```python
from build123d import *

# Parameters (mm, degrees)
F1_DEPTH = 10
F4_DEPTH = 7.5
F2_R     = 22.5
F5_DEPTH = 10.001
F2_R_2   = 40
F6_DEPTH = 5


with BuildPart() as f1:
    # F0 (on Top) → F1 (new body)
    with BuildSketch(Plane.XY):
        Polygon((43.915, 38.863247), (36.278247, 46.5), (-36.278247, 46.5), (-43.915, 38.863247), (-43.915, -46.5), (43.915, -46.5), align=None)
    extrude(amount=F1_DEPTH)

    # F3 (on face) → F4 (cut)
    with BuildSketch(Plane.XY.offset(10)):
        Polygon((-40, 3.114054), (-40, -46.500151), (-36.5154, -46.500151), (-36.5154, -9.207999), (-34, -9.207999), (-34, 3.114054), align=None)
    extrude(amount=-F4_DEPTH, mode=Mode.SUBTRACT)

    # F2 (on face) → F5 (cut, through all)
    with BuildSketch(Plane.XY.offset(10)):
        with Locations((0, 4)):
            Circle(F2_R)
    extrude(amount=-F5_DEPTH, mode=Mode.SUBTRACT)

    # F2 (on face) → F6 (cut)
    with BuildSketch(Plane.XY.offset(10)):
        with Locations((0, 4)):
            Circle(F2_R_2)
        with BuildLine():
            ThreePointArc((2, 35.686945), (31.75, 4), (2, -27.686945))
            Line((2, -27.686945), (2, -25.15))
            Line((2, -25.15), (-2, -25.15))
            Line((-2, -25.15), (-2, -27.686945))
            ThreePointArc((-2, -27.686945), (-31.75, 4), (-2, 35.686945))
            Line((-2, 35.686945), (-2, 33.15))
            Line((-2, 33.15), (2, 33.15))
            Line((2, 33.15), (2, 35.686945))
        make_face(mode=Mode.SUBTRACT)
    extrude(amount=-F6_DEPTH, mode=Mode.SUBTRACT)


solid = f1.part
```
The model under review builds one solid part; all positions refer to its coordinate system, in mm. A direction names the side the tool comes from. Coordinates: 2 decimals unless noted, no trailing zeros. Write each loop counter-clockwise with the first axis right and the second up, starting at its lowest first coordinate (ties: lowest second). Pieces come first, ordered by that corner, then holes. Notation, with made-up numbers: (12, -27.5) -> (50, -27.5) arc R5 ccw to (50, -19.5) -> close; hole circle Ø1 at (5.25, -8). An arc over 180 degrees is marked (long way). One line per item, written item: value. Start each with the question number.
Q1. Add section D-D, the plane x = -38. Give the boundary of the cut face in (y, z), then the cut area to 3 significant figures.
Q2. Add section A-A, the plane z = 8.75. Give the boundary of the cut face in (x, y) (3 decimals), then the cut area to 3 significant figures.
Q3. The part is to be moulded in two halves that separate along X. For faces 4 (the face through (-43.915, -3, 5)), 5 (the face through (1, 46.5, 5)), 6 (the face through (40.15, 42.63, 4.93)), 7 (the face through (-31.743, 3.33, 7.535)), say which applies: +X half, -X half, draft (parallel to the pull), parting line (faces both ways), or undercut.
Q4. To check wall thickness, follow probe 1 along Y at (x, z) = (0, 8.25); probe 2 along Y at (x, z) = (0, 3.5); probe 3 along X at (y, z) = (-16.5, 9) (3 decimals). State the ranges of each line that lie inside material, in increasing order.
Q5. Add section C-C, the plane y = 2. Give the boundary of the cut face in (x, z) (3 decimals).
Q6. Add section B-B, the plane x = 0. Give the boundary of the cut face in (y, z), then the cut area to 4 significant figures.
Q7. For faces 1 (the face through (-36.515, -28, 6)), 2 (the face through (-2, 34, 8)), 3 (the face through (10.382, -15.961, 5.07)), list the 3-axis set-ups (+Z, -Z, +X, -X, +Y, -Y) from which the entire face can be reached by the end or side of a thin tool; tool diameter is ignored.
Response:
1. outline: (-46.5, 0) -> (44.78, 0) -> (44.78, 10) -> (16.49, 10) -> (16.49, 5) -> (3.11, 5) -> (3.11, 2.5) -> (-46.5, 2.5) -> close
1. area: 474 mm²
2. outline: (-43.915, -46.5) -> (-40, -46.5) -> (-40, 3.114) -> (-39.99, 3.114) arc R40 cw (long way) to (-36.515, -12.329) -> (-36.515, -46.5) -> (43.915, -46.5) -> (43.915, 38.863) -> (36.278, 46.5) -> (-36.278, 46.5) -> (-43.915, 38.863) -> close; (-2, -27.687) -> (-2, -25.15) -> (2, -25.15) -> (2, -27.687) arc R31.75 ccw to (2, 35.687) -> (2, 33.15) -> (-2, 33.15) -> (-2, 35.687) arc R31.75 ccw to start; hole circle Ø45 at (0, 4)
2. area: 4,500 mm²
3. face 4: -X half
3. face 5: draft
3. face 6: +X half
3. face 7: undercut
4. probe 1: -46.5 to -36, -25.15 to -18.5, 26.5 to 33.15, 44 to 46.5
4. probe 2: -46.5 to -18.5, 26.5 to 46.5
4. probe 3: -43.915 to -40, -36.515 to -34.347, -24.245 to -9.274, 9.274 to 24.245, 34.347 to 43.915
5. outline: (-43.915, 0) -> (-22.411, 0) -> (-22.411, 10) -> (-31.687, 10) -> (-31.687, 5) -> (-34, 5) -> (-34, 2.5) -> (-40, 2.5) -> (-40, 10) -> (-43.915, 10) -> close; (22.411, 0) -> (43.915, 0) -> (43.915, 10) -> (39.95, 10) -> (39.95, 5) -> (31.687, 5) -> (31.687, 10) -> (22.411, 10) -> close
6. outline: (-46.5, 0) -> (-18.5, 0) -> (-18.5, 10) -> (-25.15, 10) -> (-25.15, 5) -> (-36, 5) -> (-36, 10) -> (-46.5, 10) -> close; (26.5, 0) -> (46.5, 0) -> (46.5, 10) -> (44, 10) -> (44, 5) -> (33.15, 5) -> (33.15, 10) -> (26.5, 10) -> close
6. area: 371.5 mm²
7. face 1: +Z, -Y
7. face 2: +Z
7. face 3: +Z, -Z
